Verification items for the finished model (mm, model axes). A direction names the side the tool comes from. Coordinates: 2 decimals unless noted, no trailing zeros. Order: outer loops, then holes, each group sorted by start corner. A loop starts at its lowest first (then second) coordinate and runs counter-clockwise, first axis right, second up. Notation, with made-up numbers: (-11, 34.5) - (14, 34.5) arc R27 cw to (14, 72.5) - close; hole circle Ø8 at (15.25, 18.5). An arc over 180 degrees is marked (long way). Answer as CSV lines item,"result". Start each with the question number.
1. Material ranges on L1, parallel to Z at x = -12, y = 7.5; L2, parallel to X at y = 1, z = -47; L3, parallel to Z at x = -3, y = 9.5, recorded low to high. Write a range as [from, to].
2. Mould release check, pull along Z, two halves, no side actions. Record for faces 4 (the cylindrical face through (-28, 1, -1)), 5 (the flat face through (50, 1, -7)), 6 (the flat face through (16.724, 0.986, -40.086)): pulls with the +Z half, pulls with the -Z half, needs draft (parallel to the pull), parting line crosses it, or undercut.
3. Section check B-B (y = 23). Record the cut outline in (x, z).
4. Section check C-C (x = -22.5). Record the cut outline in (y, z).
5. Go/stop test with flat-tipped pins: pin 1 (8 mm diameter, centred on y = 26, z = -35, fed in from +X); pin 2 (6.5 mm diameter, centred on x = -7.5, z = -7.5, fed in from +Y); pin 3 (5 mm diameter, centred on x = -19.5, y = 11, fed in from +Z); pin 4 (10 mm diameter, centred on x = 26.5, z = -26.5, fed in from -Y). Record where each tip stops, or that it passes through.
6. Section check D-D (x = 33). Record the cut outline in (y, z), and give its area (3 significant figures).
7. Set-up check for faces 1 (the cylindrical face through (48, 1, -41)), 2 (the cylindrical face through (-29, 1, -13)), 3 (the flat face through (-19, 2, -46)): record each of +Z, -Z, +X, -X, +Y, -Y from which the full face is reachable in a straight line by a thin tool's end or side.
8. Section check A-A (x = 42.5). Record the cut outline in (y, z), and give its area (3 significant figures).
from build123d import *

# Parameters (mm, degrees)
SKETCH1_R             = 2
BOSS_EXTRUDE3_DEPTH   = 30
BOSS_EXTRUDE3_2_DEPTH = 30
BOSS_EXTRUDE5_DEPTH   = 2
BOSS_EXTRUDE7_DEPTH   = 30
BOSS_EXTRUDE8_DEPTH   = 30
SKETCH6_W             = 28.26658805
SKETCH6_H             = 20
CUT_EXTRUDE2_DEPTH    = 9
SKETCH1_11_R          = 0.6
BOSS_EXTRUDE9_DEPTH   = 36
BOSS_EXTRUDE9_2_DEPTH = 36
SKETCH1_12_R          = 0.6
BOSS_EXTRUDE10_DEPTH  = 30
SKETCH8_W             = 13.05
SKETCH8_H             = 28.046654986
CUT_EXTRUDE3_DEPTH    = 7
CUT_EXTRUDE8_DEPTH    = 50
FILLET2_R             = 5
SKETCH11_W            = 12.973509336
SKETCH11_H            = 26.046654986
CUT_EXTRUDE9_DEPTH    = 52
BOSS_EXTRUDE11_DEPTH  = 2


with BuildPart() as part:
    # Sketch1 → Boss-Extrude3 (new body)
    with BuildSketch(Plane(origin=(0, 0, 0), x_dir=(1, 0, 0), z_dir=(0, 1, 0))):
        with BuildLine():
            Line((-15, 55), (-15, 0))
            Line((-15, 0), (-2.116620816, 0))
            ThreePointArc((-2.116620816, 0), (-3.706282257, 3.601240366), (-4.25, 7.5))
            ThreePointArc((-4.25, 7.5), (-3.706282257, 11.398759634), (-2.116620816, 15))
            Line((-2.116620816, 15), (-7.5, 15))
            Line((-7.5, 15), (0, 25.909090909))
            Line((0, 25.909090909), (0, 55))
            Line((0, 55), (-15, 55))
        make_face()
        with BuildLine():
            ThreePointArc((-9.5, 45), (-7.5, 47), (-5.5, 45))
            Line((-5.5, 45), (-5.5, 25))
            ThreePointArc((-5.5, 25), (-7.5, 23), (-9.5, 25))
            Line((-9.5, 25), (-9.5, 45))
        make_face(mode=Mode.SUBTRACT)
        with Locations((-7.5, 7.5)):
            Circle(SKETCH1_R, mode=Mode.SUBTRACT)
    extrude(amount=BOSS_EXTRUDE3_DEPTH)



with BuildPart() as body_2:
    # Sketch1 → Boss-Extrude3 2 (new body)
    with BuildSketch(Plane(origin=(0, 0, 0), x_dir=(1, 0, 0), z_dir=(0, 1, 0))):
        with BuildLine():
            ThreePointArc((22.116620816, 15), (23.706282257, 11.398759634), (24.25, 7.5))
            Line((24.25, 7.5), (25.5, 7.5))
            ThreePointArc((25.5, 7.5), (27.5, 9.5), (29.5, 7.5))
            Line((29.5, 7.5), (35, 7.5))
            Line((35, 7.5), (35, 55))
            Line((35, 55), (20, 55))
            Line((20, 55), (20, 25.909090909))
            Line((20, 25.909090909), (27.5, 15))
            Line((27.5, 15), (22.116620816, 15))
        make_face()
        with BuildLine():
            Line((29.5, 45), (29.5, 25))
            ThreePointArc((29.5, 25), (27.5, 23), (25.5, 25))
            Line((25.5, 25), (25.5, 45))
            ThreePointArc((25.5, 45), (27.5, 47), (29.5, 45))
        make_face(mode=Mode.SUBTRACT)
    extrude(amount=BOSS_EXTRUDE3_2_DEPTH)


with BuildPart() as part_1:
    add(part.part)

    add(body_2.part)  # Boss-Extrude5 merges body 2
    # Sketch1_6 → Boss-Extrude5 (add)
    with BuildSketch(Plane(origin=(0, 0, 0), x_dir=(1, 0, 0), z_dir=(0, 1, 0))):
        with BuildLine():
            Line((-19, 47.5), (-15, 47.5))
            Line((-15, 47.5), (-15, 55))
            Line((-15, 55), (-30, 55))
            Line((-30, 55), (-30, 47.5))
            Line((-30, 47.5), (-26, 47.5))
            ThreePointArc((-26, 47.5), (-22.5, 51), (-19, 47.5))
        make_face()
        with BuildLine():
            Line((-30, 40), (-15, 40))
            Line((-15, 40), (-15, 47.5))
            Line((-15, 47.5), (-19, 47.5))
            ThreePointArc((-19, 47.5), (-22.5, 44), (-26, 47.5))
            Line((-26, 47.5), (-30, 47.5))
            Line((-30, 47.5), (-30, 40))
        make_face()
        with BuildLine():
            Line((35, 55), (35, 47.5))
            Line((35, 47.5), (39, 47.5))
            ThreePointArc((39, 47.5), (42.5, 51), (46, 47.5))
            Line((46, 47.5), (50, 47.5))
            Line((50, 47.5), (50, 55))
            Line((50, 55), (35, 55))
        make_face()
        with BuildLine():
            Line((35, 47.5), (35, 40))
            Line((35, 40), (50, 40))
            Line((50, 40), (50, 47.5))
            Line((50, 47.5), (46, 47.5))
            ThreePointArc((46, 47.5), (42.5, 44), (39, 47.5))
            Line((39, 47.5), (35, 47.5))
        make_face()
        with BuildLine():
            Line((35, 15), (35, 7.5))
            Line((35, 7.5), (39, 7.5))
            ThreePointArc((39, 7.5), (42.5, 11), (46, 7.5))
            Line((46, 7.5), (50, 7.5))
            Line((50, 7.5), (50, 15))
            Line((50, 15), (39.7, 15))
            Line((39.7, 15), (35, 15))
        make_face()
        with BuildLine():
            Line((35, 7.5), (35, 0))
            Line((35, 0), (50, 0))
            Line((50, 0), (50, 7.5))
            Line((50, 7.5), (46, 7.5))
            ThreePointArc((46, 7.5), (42.5, 4), (39, 7.5))
            Line((39, 7.5), (35, 7.5))
        make_face()
        with BuildLine():
            Line((-19, 7.5), (-15, 7.5))
            Line((-15, 7.5), (-15, 15))
            Line((-15, 15), (-30, 15))
            Line((-30, 15), (-30, 7.5))
            Line((-30, 7.5), (-26, 7.5))
            ThreePointArc((-26, 7.5), (-22.5, 11), (-19, 7.5))
        make_face()
        with BuildLine():
            Line((-30, 0), (-15, 0))
            Line((-15, 0), (-15, 7.5))
            Line((-15, 7.5), (-19, 7.5))
            ThreePointArc((-19, 7.5), (-22.5, 4), (-26, 7.5))
            Line((-26, 7.5), (-30, 7.5))
            Line((-30, 7.5), (-30, 0))
        make_face()
    extrude(amount=BOSS_EXTRUDE5_DEPTH)

    # Sketch1_8 → Boss-Extrude7 (add)
    with BuildSketch(Plane(origin=(0, 0, 0), x_dir=(1, 0, 0), z_dir=(0, 1, 0))):
        with BuildLine():
            Line((-2.116620816, 0), (-4.133294025, 0))
            ThreePointArc((-4.133294025, 0), (1.753788749, -6.211309201), (10, -8.5))
            ThreePointArc((10, -8.5), (18.246211251, -6.211309201), (24.133294025, 0))
            Line((24.133294025, 0), (22.116620816, 0))
            ThreePointArc((22.116620816, 0), (10, -6.75), (-2.116620816, 0))
        make_face()
    extrude(amount=BOSS_EXTRUDE7_DEPTH)

    # Sketch1_9 → Boss-Extrude8 (add)
    with BuildSketch(Plane(origin=(0, 0, 0), x_dir=(1, 0, 0), z_dir=(0, 1, 0))):
        with BuildLine():
            ThreePointArc((24.25, 7.5), (23.706282257, 3.601240366), (22.116620816, 0))
            Line((22.116620816, 0), (24.133294025, 0))
            Line((24.133294025, 0), (35, 0))
            Line((35, 0), (35, 7.5))
            Line((35, 7.5), (29.5, 7.5))
            ThreePointArc((29.5, 7.5), (27.5, 5.5), (25.5, 7.5))
            Line((25.5, 7.5), (24.25, 7.5))
        make_face()
    extrude(amount=BOSS_EXTRUDE8_DEPTH)

    # Sketch6 → Cut-Extrude2 (cut)
    with BuildSketch(Plane.XY):
        with Locations((10, 20)):
            Rectangle(SKETCH6_W, SKETCH6_H)
    extrude(amount=CUT_EXTRUDE2_DEPTH, mode=Mode.SUBTRACT)



with BuildPart() as body_2_2:
    # Sketch1_11 → Boss-Extrude9 (new body)
    with BuildSketch(Plane(origin=(0, 0, 0), x_dir=(1, 0, 0), z_dir=(0, 1, 0))):
        with Locations((38.4, 25)):
            Circle(SKETCH1_11_R)
    extrude(amount=BOSS_EXTRUDE9_DEPTH)


with BuildPart() as body_3:
    # Sketch1_11 → Boss-Extrude9 2 (new body)
    with BuildSketch(Plane(origin=(0, 0, 0), x_dir=(1, 0, 0), z_dir=(0, 1, 0))):
        with Locations((44.9, 25)):
            Circle(SKETCH1_11_R)
    extrude(amount=BOSS_EXTRUDE9_2_DEPTH)


with BuildPart() as part_2:
    add(part_1.part)

    add(body_2_2.part)  # Boss-Extrude10 merges body 2 2

    add(body_3.part)  # Boss-Extrude10 merges body 3
    # Sketch1_12 → Boss-Extrude10 (add)
    with BuildSketch(Plane(origin=(0, 0, 0), x_dir=(1, 0, 0), z_dir=(0, 1, 0))):
        Polygon((35, 26.5), (35, 20), (48.05, 20), (48.05, 26.5), (38.4, 26.5), align=None)
        with BuildLine():
            ThreePointArc((39, 25), (37.975735931, 24.575735931), (38.4, 25.6))
            ThreePointArc((38.4, 25.6), (38.824264069, 25.424264069), (39, 25))
        make_face(mode=Mode.SUBTRACT)
        with Locations((44.9, 25)):
            Circle(SKETCH1_12_R, mode=Mode.SUBTRACT)
    extrude(amount=BOSS_EXTRUDE10_DEPTH)

    # Sketch8 → Cut-Extrude3 (cut)
    with BuildSketch(Plane.XY.offset(-20)):
        with Locations((41.525, 14.023327493)):
            Rectangle(SKETCH8_W, SKETCH8_H)
    extrude(amount=-CUT_EXTRUDE3_DEPTH, mode=Mode.SUBTRACT)

    # Sketch10 → Cut-Extrude8 (cut)
    with BuildSketch(Plane(origin=(35, 0, 0), x_dir=(0, 0, -1), z_dir=(1, 0, 0))):
        Polygon((15, 2), (15, 0), (40, 0), (47.5, 0), (47.5, 28.046654986), (15, 28.046654986), align=None)
    extrude(amount=-CUT_EXTRUDE8_DEPTH, mode=Mode.SUBTRACT)

    # Fillet2
    fillet2_edges = [part_2.edges().sort_by_distance(p)[0] for p in [
        (-30, 1, -15),
        (35, 1, -40),
        (50, 1, -40),
        (50, 1, -55),
        (50, 1, 0),
        (50, 1, -15),
        (-15, 1, -40),
        (-30, 1, 0),
        (-30, 1, -40),
        (-30, 1, -55),
    ]]
    fillet(fillet2_edges, radius=FILLET2_R)

    # Sketch11 → Cut-Extrude9 (cut)
    with BuildSketch(Plane(origin=(35, 0, 0), x_dir=(0, 0, -1), z_dir=(1, 0, 0))):
        with Locations((8.513245332, 15.023327493)):
            Rectangle(SKETCH11_W, SKETCH11_H)
    extrude(amount=-CUT_EXTRUDE9_DEPTH, mode=Mode.SUBTRACT)

    # Sketch1_13 → Boss-Extrude11 (add)
    with BuildSketch(Plane(origin=(0, 0, 0), x_dir=(1, 0, 0), z_dir=(0, 1, 0))):
        with BuildLine():
            Line((-7.5, 15), (-2.116620816, 15))
            ThreePointArc((-2.116620816, 15), (-1.137525113, 16.389208872), (0, 17.651970252))
            Line((0, 17.651970252), (0, 25.909090909))
            Line((0, 25.909090909), (-7.5, 15))
        make_face()
        with BuildLine():
            Line((0, 25.909090909), (0, 17.651970252))
            ThreePointArc((0, 17.651970252), (1.621777227, 19.02683318), (3.43006352, 20.145095281))
            Line((3.43006352, 20.145095281), (10, 30))
            Line((10, 30), (6.461538462, 35.307692308))
            Line((6.461538462, 35.307692308), (0, 25.909090909))
        make_face()
        Polygon((10, 40.454545455), (6.461538462, 35.307692308), (10, 30), (13.538461538, 35.307692308), align=None)
        Polygon((20, 55), (10, 40.454545455), (13.538461538, 35.307692308), (20, 45), align=None)
        Polygon((0, 55), (0, 45), (6.461538462, 35.307692308), (10, 40.454545455), align=None)
        with BuildLine():
            ThreePointArc((16.56993648, 20.145095281), (18.378222773, 19.02683318), (20, 17.651970252))
            Line((20, 17.651970252), (20, 25.909090909))
            Line((20, 25.909090909), (13.538461538, 35.307692308))
            Line((13.538461538, 35.307692308), (10, 30))
            Line((10, 30), (16.56993648, 20.145095281))
        make_face()
        with BuildLine():
            ThreePointArc((20, 17.651970252), (21.137525113, 16.389208872), (22.116620816, 15))
            Line((22.116620816, 15), (27.5, 15))
            Line((27.5, 15), (20, 25.909090909))
            Line((20, 25.909090909), (20, 17.651970252))
        make_face()
    extrude(amount=BOSS_EXTRUDE11_DEPTH)


solid = part_2.part
Evaluation:
1,L1,"z = [-55, -47.5], [-2.03, 0]"
1,L2,"x = [-30, -25.96], [-19.04, -15], [0, 5.5], [14.5, 20], [35, 39.04], [45.96, 50]"
1,L3,"z = [-55, -47.5], [-1.66, 1.83]"
2,face 4,"pulls with the +Z half"
2,face 5,"needs draft"
2,face 6,"undercut"
3,outline,"(-15, -55) - (0, -55) - (0, -47.5) - (-15, -47.5) - close; (-15, -2.03) - (-3.16, -2.03) arc R14.25 cw to (-2.12, 0) - (-15, 0) - close; (20, -55) - (35, -55) - (35, -47.5) - (20, -47.5) - close; (22.12, 0) arc R14.25 cw to (23.16, -2.03) - (35, -2.03) - (35, 0) - close"
4,outline,"(0, -55) - (2, -55) - (2, -51) - (0, -51) - close; (0, -44) - (2, -44) - (2, -40) - (0, -40) - close; (0, -15) - (2, -15) - (2, -11) - (0, -11) - close; (0, -4) - (2, -4) - (2, 0) - (0, 0) - close"
5,pin 1,"stops at x = 35"
5,pin 2,"stops at y = 30"
5,pin 3,"passes through"
5,pin 4,"stops at y = 28.05"
6,outline,"(0, -55) - (30, -55) - (30, 0) - (0, 0) - (0, -15) - (2, -15) - (2, -2.03) - (28.05, -2.03) - (28.05, -47.5) - (0, -47.5) - close"
6,area,"401 mm²"
7,face 1,"+X, +Y, -Y"
7,face 2,"-X, +Y, -Y"
7,face 3,"+Z, -Z, -X, +Y"
8,outline,"(0, -55) - (2, -55) - (2, -51) - (0, -51) - close; (0, -44) - (2, -44) - (2, -40) - (0, -40) - close; (0, -15) - (2, -15) - (2, -11) - (0, -11) - close; (0, -4) - (2, -4) - (2, 0) - (0, 0) - close; (28.05, -26.5) - (30, -26.5) - (30, -20) - (28.05, -20) - close"
8,area,"44.7 mm²"
